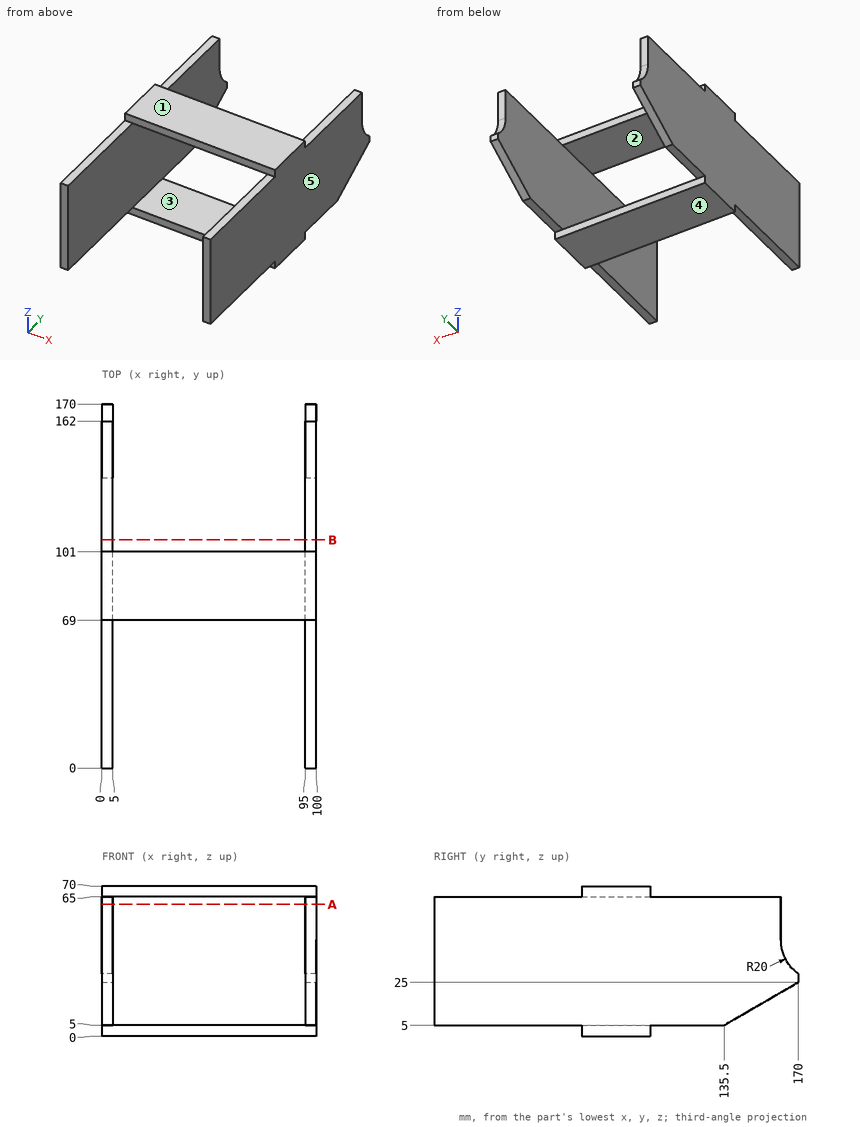
Source: three-view drawing plus pictorial views. Frame: mm from the lowest corner of the part. A direction names the side the tool comes from. Give positions to 0.01 mm unless a question says otherwise; leave off trailing zeros. Write each loop counter-clockwise with the first axis right and the second up, starting at its lowest first coordinate (ties: lowest second). Pieces come first, ordered by that corner, then holes. Notation, with made-up numbers: (-13.5, 44) - (3.5, 44) arc R34 ccw to (3.5, 83) - close; hole circle Ø7 at (65, 87). An arc over 180 degrees is marked (long way). Write item = value, one per line. Start each with the question number.
Q1. Cut plane B-B, the plane y = 106.5. Return loops of the section in (x, z).
Q2. Pin query (flat end, axial travel): pin 1 Ø4 at (x, z) = (52.5, 1.5) entering from -Y; pin 2 Ø2.5 at (x, y) = (2.5, 25.5) entering from +Z; pin 3 Ø2.5 at (x, y) = (1.5, 48.5) entering from -Z. Return the tip coordinate at first contact, or that it passes through.
Q3. Draft query along X for the marked faces 3, 4 and 5. Return one class per face: +X half, -X half, draft (parallel to the pull), parting line (faces both ways), or undercut.
Q4. Reachability of the marked faces 1 and 2 from +Z, -Z, +X, -X, +Y, -Y: full face, straight path, thin tool, end or side. Return the list, or none.
Q5. Cut plane A-A, the plane z = 61.5. Return loops of the section in (x, y).
Q6. Material intervals for probe 1 along X at (y, z) = (75, 21.5); probe 2 along Z at (x, y) = (21.5, 93); probe 3 along Y at (x, z) = (96.5, 39.5), sorted ascending.
Computed values:
q1.outline = (0, 5) - (5, 5) - (5, 65) - (0, 65) - close; (95, 5) - (100, 5) - (100, 65) - (95, 65) - close
q2.pin_1 = 69
q2.pin_2 = 65
q2.pin_3 = 5
q3.face_3 = undercut
q3.face_4 = draft
q3.face_5 = +X half
q4.face_1 = +Z, +X, -X, +Y, -Y
q4.face_2 = +Y, -Y
q5.outline = (0, 0) - (5, 0) - (5, 162) - (0, 162) - close; (95, 0) - (100, 0) - (100, 162) - (95, 162) - close
q6.probe_1 = 0 to 5, 95 to 100
q6.probe_2 = 0 to 5, 65 to 70
q6.probe_3 = 0 to 162.77
